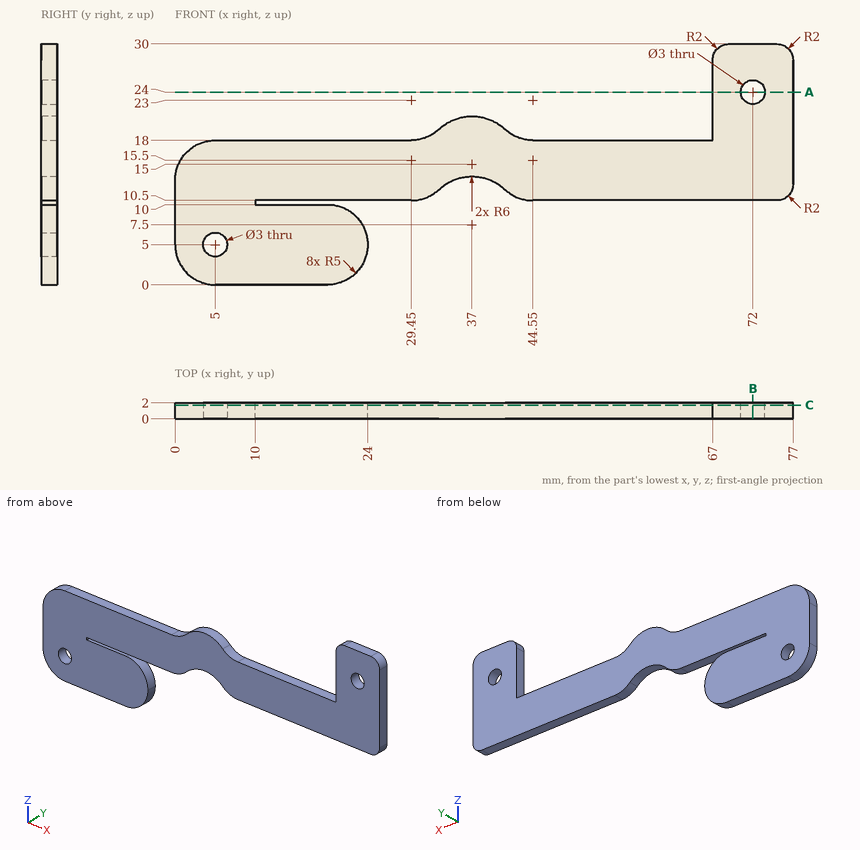
Part print with two shaded views. Sizes in mm from the minimum x, y, z corner. Give positions to 0.01 mm unless a question says otherwise; leave off trailing zeros. Order: outer loops, then holes, each group sorted by start corner. A loop starts at its lowest first (then second) coordinate and runs counter-clockwise, first axis right, second up.
(1) Flat gauge pins, fed straight in: pin 1 (3 mm diameter, centred on x = 29, z = 21, fed in from -Y); pin 2 (0.6 mm diameter, centred on y = 1, z = 10.5, fed in from +X); pin 3 (0.6 mm diameter, centred on x = 22, y = 1.5, fed in from +Z). Where does each tip first touch, or does it go through?
(2) Saw through at C-C, the plane y = 1.7. State how many separate pieces and enclosed holes the cut face has, then the cut area to 3 significant figures.
(3) Drill centre lines: L1, parallel to Z at x = 72, y = 0.7; L2, parallel to Z at x = 16.5, y = 1.3; L3, parallel to X at y = 1.55, z = 24. Where is each one in solid material? Low to high.
(4) Saw through at A-A, the plane z = 24. Give the cut face in (x, y), then the cut area to 3 significant figures.
(5) Saw through at B-B, the plane x = 72. Give the cut face in (y, z), then the cut area to 3 significant figures.
Results found:
1. pin 1: passes through
1. pin 2: stops at x = 76.05
1. pin 3: stops at z = 18
2. separate pieces: 1
2. enclosed holes: 2
2. area: 904 mm2
3. L1: z = 10.5 to 22.5, 25.5 to 30
3. L2: z = 0 to 10, 10.5 to 18
3. L3: x = 67 to 70.5, 73.5 to 77
4. outline: (67, 0) - (70.5, 0) - (70.5, 2) - (67, 2) - close; (73.5, 0) - (77, 0) - (77, 2) - (73.5, 2) - close
4. area: 14.0 mm2
5. outline: (0, 10.5) - (2, 10.5) - (2, 22.5) - (0, 22.5) - close; (0, 25.5) - (2, 25.5) - (2, 30) - (0, 30) - close
5. area: 33.0 mm2
